Autodesk Inventor part; units mm, degrees
ref_plane "Начальная плоскость" through (0, 0, 10) normal (0, 0, 1) x (1, 0, 0)
ref_plane "Конечная плоскость" through (0, 0, 320) normal (0, 0, 1) x (1, 0, 0)
ref_plane "РабПлоскость4" through (-255, -8.5, 320) normal (0, 0, 1) x (1, 0, 0)
ref_plane "Начальная плоскость" through (0, 0, 10) normal (0, 0, 1) x (1, 0, 0)
ref_plane "Конечная плоскость" through (0, 0, 320) normal (0, 0, 1) x (1, 0, 0)
sketch "Эскиз" plane through (0, 0, 0) normal (0, 0, 1) x (1, 0, 0)
  line L0 (-14.4349, 0) -> (14.4349, 0)
  line L1 (0, -14) -> (0, 14)
  line L2 (0, 0) -> (7.5, 7.5) construction
  circle A0 centre (7.5, 7.5) radius 1.65 construction
  line L3 (5.85, 9.15) -> (9.15, 9.15)
  line L4 (9.15, 9.15) -> (9.15, 5.85)
  line L5 (9.15, 5.85) -> (5.85, 5.85)
  line L6 (5.85, 5.85) -> (5.85, 9.15)
  line L7 (3.235, 8.1636) -> (4.72, 9.9636)
  line L8 (4.7971, 10) -> (8.5, 10)
  line L9 (3.3121, 8) -> (4.95, 8)
  line L10 (4.95, 8) -> (4.95, 5.7985)
  line L11 (4.95, 5.7985) -> (2.6515, 3.5)
  line L12 (0, 3.5) -> (2.6515, 3.5)
  circle A1 centre (0, 0) radius 2.5
  line L13 (8.1636, 3.235) -> (9.9636, 4.72)
  line L14 (10, 4.7971) -> (10, 8.5)
  line L15 (8, 3.3121) -> (8, 4.95)
  line L16 (8, 4.95) -> (5.7985, 4.95)
  line L17 (5.7985, 4.95) -> (3.5, 2.6515)
  line L18 (3.5, 0) -> (3.5, 2.6515)
  arc A2 (10, 8.5) -> (8.5, 10) centre (8.5, 8.5) ccw
  line L19 (0, 0) -> (-7.5, 7.5) construction
  circle A3 centre (-7.5, 7.5) radius 1.65 construction
  line L20 (-5.85, 9.15) -> (-9.15, 9.15)
  line L21 (-9.15, 9.15) -> (-9.15, 5.85)
  line L22 (-9.15, 5.85) -> (-5.85, 5.85)
  line L23 (-5.85, 5.85) -> (-5.85, 9.15)
  line L24 (-3.235, 8.1636) -> (-4.72, 9.9636)
  line L25 (-4.7971, 10) -> (-8.5, 10)
  line L26 (-3.3121, 8) -> (-4.95, 8)
  line L27 (-4.95, 8) -> (-4.95, 5.7985)
  line L28 (-4.95, 5.7985) -> (-2.6515, 3.5)
  line L29 (0, 3.5) -> (-2.6515, 3.5)
  line L30 (-3.5, 0) -> (-3.5, 2.6515)
  line L31 (-5.7985, 4.95) -> (-3.5, 2.6515)
  line L32 (-8, 4.95) -> (-5.7985, 4.95)
  line L33 (-8, 3.3121) -> (-8, 4.95)
  line L34 (-8.1636, 3.235) -> (-9.9636, 4.72)
  line L35 (-10, 4.7971) -> (-10, 8.5)
  arc A4 (-8.5, 10) -> (-10, 8.5) centre (-8.5, 8.5) ccw
  line L36 (0, 14) -> (0, -14)
  line L37 (0, 0) -> (7.5, -7.5) construction
  circle A5 centre (7.5, -7.5) radius 1.65 construction
  line L38 (5.85, -9.15) -> (9.15, -9.15)
  line L39 (9.15, -9.15) -> (9.15, -5.85)
  line L40 (9.15, -5.85) -> (5.85, -5.85)
  line L41 (5.85, -5.85) -> (5.85, -9.15)
  line L42 (3.235, -8.1636) -> (4.72, -9.9636)
  line L43 (4.7971, -10) -> (8.5, -10)
  line L44 (3.3121, -8) -> (4.95, -8)
  line L45 (4.95, -8) -> (4.95, -5.7985)
  line L46 (4.95, -5.7985) -> (2.6515, -3.5)
  line L47 (0, -3.5) -> (2.6515, -3.5)
  line L48 (3.5, 0) -> (3.5, -2.6515)
  line L49 (5.7985, -4.95) -> (3.5, -2.6515)
  line L50 (8, -4.95) -> (5.7985, -4.95)
  line L51 (8, -3.3121) -> (8, -4.95)
  line L52 (8.1636, -3.235) -> (9.9636, -4.72)
  line L53 (10, -4.7971) -> (10, -8.5)
  arc A6 (8.5, -10) -> (10, -8.5) centre (8.5, -8.5) ccw
  line L54 (0, 0) -> (-7.5, -7.5) construction
  line L55 (-4.95, -8) -> (-4.95, -5.7985)
  line L56 (-3.3121, -8) -> (-4.95, -8)
  line L57 (-5.7985, -4.95) -> (-3.5, -2.6515)
  line L58 (-4.95, -5.7985) -> (-2.6515, -3.5)
  line L59 (-3.5, 0) -> (-3.5, -2.6515)
  line L60 (0, -3.5) -> (-2.6515, -3.5)
  circle A7 centre (-7.5, -7.5) radius 1.65 construction
  line L61 (-5.85, -5.85) -> (-5.85, -9.15)
  line L62 (-5.85, -9.15) -> (-9.15, -9.15)
  line L63 (-9.15, -9.15) -> (-9.15, -5.85)
  line L64 (-9.15, -5.85) -> (-5.85, -5.85)
  line L65 (-3.235, -8.1636) -> (-4.72, -9.9636)
  line L66 (-8, -4.95) -> (-5.7985, -4.95)
  line L67 (-8, -3.3121) -> (-8, -4.95)
  line L68 (-8.1636, -3.235) -> (-9.9636, -4.72)
  line L69 (-4.7971, -10) -> (-8.5, -10)
  line L70 (-10, -4.7971) -> (-10, -8.5)
  arc A8 (-10, -8.5) -> (-8.5, -10) centre (-8.5, -8.5) ccw
  arc A9 (3.235, 8.1636) -> (3.3121, 8) centre (3.3121, 8.1) ccw
  arc A10 (4.7971, 10) -> (4.72, 9.9636) centre (4.7971, 9.9) ccw
  arc A11 (8, 3.3121) -> (8.1636, 3.235) centre (8.1, 3.3121) ccw
  arc A12 (9.9636, 4.72) -> (10, 4.7971) centre (9.9, 4.7971) ccw
  arc A13 (-3.3121, 8) -> (-3.235, 8.1636) centre (-3.3121, 8.1) ccw
  arc A14 (-4.72, 9.9636) -> (-4.7971, 10) centre (-4.7971, 9.9) ccw
  arc A15 (-8.1636, 3.235) -> (-8, 3.3121) centre (-8.1, 3.3121) ccw
  arc A16 (-10, 4.7971) -> (-9.9636, 4.72) centre (-9.9, 4.7971) ccw
  arc A17 (-8, -3.3121) -> (-8.1636, -3.235) centre (-8.1, -3.3121) ccw
  arc A18 (-9.9636, -4.72) -> (-10, -4.7971) centre (-9.9, -4.7971) ccw
  arc A19 (-3.235, -8.1636) -> (-3.3121, -8) centre (-3.3121, -8.1) ccw
  arc A20 (-4.7971, -10) -> (-4.72, -9.9636) centre (-4.7971, -9.9) ccw
  arc A21 (4.72, -9.9636) -> (4.7971, -10) centre (4.7971, -9.9) ccw
  arc A22 (3.3121, -8) -> (3.235, -8.1636) centre (3.3121, -8.1) ccw
  arc A23 (8.1636, -3.235) -> (8, -3.3121) centre (8.1, -3.3121) ccw
  arc A24 (10, -4.7971) -> (9.9636, -4.72) centre (9.9, -4.7971) ccw
  point P0 (3.1, 8)
  point P1 (4.75, 10)
  point P2 (7.5, 9.15)
  point P3 (8, 3.1)
  point P4 (10, 4.75)
  point P5 (7.5, 5.85)
  point P6 (9.15, 7.5)
  point P7 (-3.1, 8)
  point P8 (-4.75, 10)
  point P9 (-7.5, 9.15)
  point P10 (-8, 3.1)
  point P11 (-10, 4.75)
  point P12 (-7.5, 5.85)
  point P13 (-9.15, 7.5)
  point P14 (3.1, -8)
  point P15 (4.75, -10)
  point P16 (7.5, -9.15)
  point P17 (8, -3.1)
  point P18 (10, -4.75)
  point P19 (7.5, -5.85)
  point P20 (9.15, -7.5)
  point P21 (-3.1, -8)
  point P22 (-7.5, -5.85)
  point P23 (-7.5, -9.15)
  point P24 (-9.15, -7.5)
  point P25 (-4.75, -10)
  point P26 (-8, -3.1)
  point P27 (-10, -4.75)
  dimension "d0" = 45
  dimension "d1" = 3.3
  dimension "d2" = 1.5
  dimension "d3" = 1.2
  dimension "d4" = 5
  dimension "d5" = 6.5
  dimension "d6" = 15
  dimension "d7" = 20
  dimension "d8" = 9.9
  dimension "d9" = 9.5
  dimension "d10" = 6.2
  dimension "d11" = 2
  dimension "d18" = 0.1
  dimension "d19" = 0.1
extrude "Тело" add sketch "Эскиз" along normal up to surface (310 mm away) from surface at 10 contours A1 L1 L12 L11 L10 L9 A9 L7 A10 L8 A2 L14 A12 L13 A11 L15 L16 L17 L18 L0 | L0 L48 L49 L50 L51 A23 L52 A24 L53 A6 L43 A21 L42 A22 L44 L45 L46 L47 L1 A1 | A1 L0 L30 L31 L32 L33 A15 L34 A16 L35 A4 L25 A14 L24 A13 L26 L27 L28 L29 L1 | L1 L60 L58 L55 L56 A19 L65 A20 L69 A8 L70 A18 L68 A17 L67 L66 L57 L59 L0 A1
sketch "Эскиз2" plane through (0, 0, 0) normal (0, 0, 1) x (1, 0, 0)
  line L0 (0, 0) -> (10, 0)
ref_plane "РабПлоскость3" through (0, 0, 0) normal (0, -1, 0) x (1, 0, 0)
sketch "Эскиз3" plane through (0, 0, 0) normal (0, -1, 0) x (1, 0, 0)
  line L0 (-2, 10) -> (12, 10)
  line L1 (-2, 320) -> (12, 320)
  dimension "d25" = 310
ref_plane "РабПлоскость4" through (-255, -8.5, 320) normal (0, 0, 1) x (1, 0, 0)
split "Разделение1" plane through (-255, -8.5, 320) removes the side toward (0, 0, 1)
ref_plane "РабПлоскость5" through (-300, 8.5, 10) normal (0, 0, -1) x (-1, 0, 0)
split "Разделение2" plane through (-300, 8.5, 10) removes the side toward (0, 0, -1)
properties part number "короткая палка" material "Алюминий 6061"
The listing builds one solid part. Answer for the finished solid, in the listing's coordinates (mm). A direction names the side the tool comes from. Round coordinates to 2 decimals unless told otherwise and drop trailing zeros. Loops run counter-clockwise (first coordinate to the right, second up) from the corner with the lowest first, then second, coordinate; pieces in that order, holes last. Notation, with made-up numbers: M -16,4.5 L 11,4.5 A30 ccw 11,32.5 Z; hole C -9.75,56.5 d7. An arc over 180 degrees is marked long. Return JSON: item names as keys, results as strings.
Q1. Find section A-A, the plane y = 0. Determine the outline of the cut face in (x, z).
Results list:
{"outline": "M -3.5,10 L -2.5,10 L -2.5,320 L -3.5,320 Z; M 2.5,10 L 3.5,10 L 3.5,320 L 2.5,320 Z"}
Q2. Find section C-C, the plane z = 150. State how many separate pieces and enclosed holes the cut face has, plus the area to 3 significant figures.
Results list:
{"separate pieces": "1", "enclosed holes": "5", "area": "115 mm2"}
Q3. Find the intervals of material crossed by line 1 along X through (y, z) = (-8.5, 268.5); line 2 along Y through (x, z) = (0, 176), in increasing order. Write a range as from..to.
Results list:
{"line 1": "x = -10..-9.15, -5.85..-3.51, 3.51..5.85, 9.15..10", "line 2": "y = -3.5..-2.5, 2.5..3.5"}
Q4. The mould has two halves that part along X. Classify faces 4 (the face through (3.5, 0, 163)), 5 (the face through (0, -3.5, 163)), 6 (the face through (0, -3, 10)): released by +X, released by -X, zero draft, split by the parting line, or undercut.
Results list:
{"face 4": "released by +X", "face 5": "undercut", "face 6": "zero draft"}
Q5. Each of these flat-tipped pins is pushed along its axis until it touches: pin 1 Ø6 at (y, z) = (1.5, 56) entering from +X; pin 2 Ø3 at (x, y) = (-6.5, -2.5) entering from +Z; pin 3 Ø6 at (x, z) = (1.5, 143) entering from +Y. Where does it stop, or does it pass through?
Results list:
{"pin 1": "stops at x = 9.7", "pin 2": "passes through", "pin 3": "stops at y = 9.7"}
Q6. Which of the six approach directions +Z, -Z, +X, -X, +Y, -Y give full straight-line access (tool end or side, diameter ignored) to faces 1 (the face through (-0.54, 2.44, 162.83)), 2 (the face through (0, 3.5, 163)), 3 (the face through (-3.5, 0, 163))?
Results list:
{"face 1": "+Z, -Z", "face 2": "+Z, -Z, +Y", "face 3": "+Z, -Z, -X"}
